Check sheet for the drawn part. Datum: minimum x, y, z corner. Units: mm. Give positions to 0.01 mm unless a question says otherwise; leave off trailing zeros. Write each loop counter-clockwise with the first axis right and the second up, starting at its lowest first coordinate (ties: lowest second). Pieces come first, ordered by that corner, then holes. Notation, with made-up numbers: (48, 39) -> (100, 39) arc R19 cw to (100, 52) -> close; hole circle Ø8 at (-8.75, -17). An arc over 180 degrees is marked (long way). Answer as CSV lines item,"result". Start each with the question number.
1) Sectioned sample at C-C on x = 62. Record the cut outline in (y, z).
2) Gauge pin test, flat ends, axial feed: pin 1 Ø1 at (y, z) = (13, 2.5) entering from -X; pin 2 Ø4 at (x, y) = (54.95, 8.32) entering from -Z. Record the tip position at first contact, or that the pin passes through.
3) Mould release check, pull along X, two halves, no side actions. Record for the marked faces 1, 2 and 3: released by +X, released by -X, zero draft, split by the parting line, or undercut.
4) Material ranges on L1, parallel to X at y = 8.5, z = 2 (1 decimal); L2, parallel to X at y = 10.25, z = 3.2 (1 decimal); L3, parallel to X at y = 9.75, z = 4.1 (1 decimal), recorded low to high.
5) Sectioned sample at D-D on y = 14.25. Record the cut outline in (x, z), and give its area (3 significant figures).
6) Sectioned sample at A-A on y = 9.5. Record the cut outline in (x, z) (1 decimal).
7) Sectioned sample at B-B on z = 3.05. Give the number of separate pieces and of enclosed holes in the cut face, and give its area (3 significant figures).
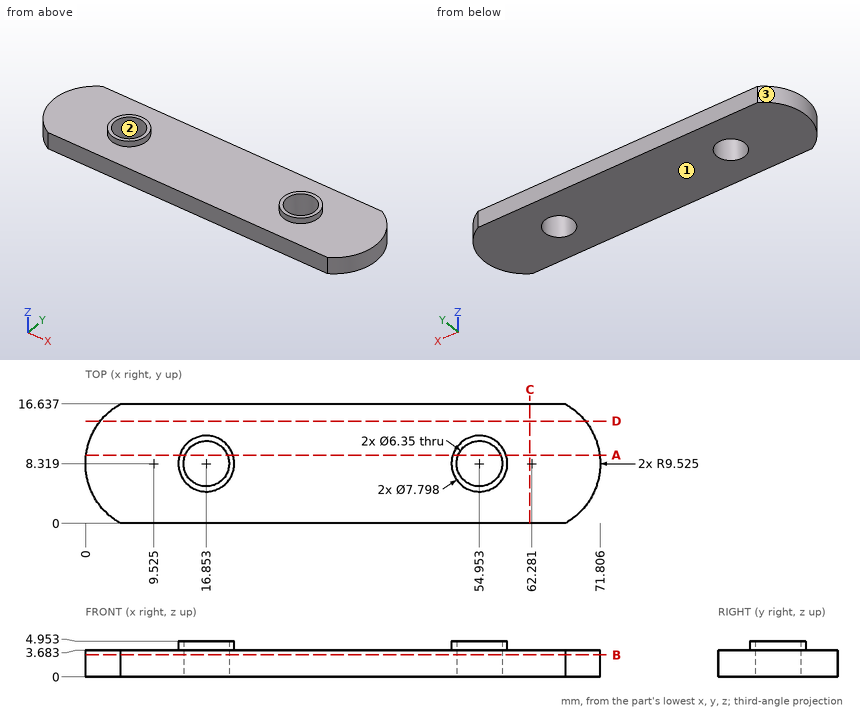
Ans:
1,outline,"(0, 0) -> (16.64, 0) -> (16.64, 3.68) -> (0, 3.68) -> close"
2,pin 1,"stops at x = 0.97"
2,pin 2,"passes through"
3,face 1,"zero draft"
3,face 2,"undercut"
3,face 3,"released by -X"
4,L1,"x = 0 to 13.7, 20 to 51.8, 58.1 to 71.8"
4,L2,"x = 0.2 to 14.3, 19.4 to 52.4, 57.5 to 71.6"
4,L3,"x = 13.2 to 14, 19.7 to 20.5, 51.3 to 52.1, 57.8 to 58.6"
5,outline,"(2.07, 0) -> (69.73, 0) -> (69.73, 3.68) -> (2.07, 3.68) -> close"
5,area,"249 mm²"
6,outline,"(0.1, 0) -> (13.9, 0) -> (13.9, 5) -> (13.1, 5) -> (13.1, 3.7) -> (0.1, 3.7) -> close; (19.8, 0) -> (52, 0) -> (52, 5) -> (51.2, 5) -> (51.2, 3.7) -> (20.6, 3.7) -> (20.6, 5) -> (19.8, 5) -> close; (57.9, 0) -> (71.7, 0) -> (71.7, 3.7) -> (58.7, 3.7) -> (58.7, 5) -> (57.9, 5) -> close"
7,separate pieces,"1"
7,enclosed holes,"2"
7,area,"1,080 mm²"
